Can you work these out from the model? Positions are in its coordinate system, mm. A direction names the side the tool comes from. Coordinates: 2 decimals unless noted, no trailing zeros. Loops run counter-clockwise (first coordinate to the right, second up) from the corner with the lowest first, then second, coordinate; pieces in that order, holes last. Notation, with made-up numbers: (17, 73.25) -> (34, 73.25) arc R20 cw to (34, 77.25) -> close; hole circle Ø7 at (3, -18). An arc over 180 degrees is marked (long way). Use one line per item in the form item = value. Start each with the question number.
(1) Imagine slicing it at A-A (y = -17.25). List the corners of the cut face in (x, z) for me (3 decimals), plus the area to 3 significant figures.
(2) Thinking about a two-plate mould opening in Z: for faces 5 (the flat face through (139.7, -9, 77)), 6 (the flat face through (129, -10, 104.775)), 7 (the flat face through (130, -10, 50.8)), which applies, released by +Z, released by -Z, zero draft, split by the parting line, or undercut?
(3) Imagine slicing it at C-C (z = 121). List the corners of the cut face in (x, y) for me (3 decimals), plus the area to 3 significant figures.
(4) I'm going to push flat-ended pins straight in: pin 1 (1 mm diameter, centred on y = -13.5, z = 128, fed in from +X) (3 decimals); pin 2 (9.5 mm diameter, centred on x = 131.5, y = -10, fed in from +Z) (3 decimals); pin 3 (5 mm diameter, centred on y = -15.5, z = 34, fed in from -X). Where does each tip first touch, or does it pass through?
(5) I need wall thicknesses on line 1 (X direction, y = -14.75, z = 110.5) (3 decimals); line 2 (X direction, y = -3.75, z = 34). Which ranges of each line are inside material? Lowest first, please. Write a range as [from, to].
(6) Imagine slicing it at B-B (x = 130.5). List the corners of the cut face in (y, z) for me (3 decimals).
(7) On a 3-axis mill with a long thin cutter (end or side, diameter ignored), from which of +Z, -Z, +X, -X, +Y, -Y can I reach the whole of each face in a straight line? I mean faces 1 (the flat face through (130.31, -9.66, 25.04)), 2 (the flat face through (22.225, -10, 128)), 3 (the flat face through (117.475, -10, 128)), 4 (the flat face through (9.39, -9.66, 25.04)). Say none if no direction works.
```python
from build123d import *

# Parameters (mm, degrees)
F0_W     = 139.7
F0_H     = 152.4
F1_DEPTH = 19.05
F2_W     = 22.225
F2_H     = 47.625
F3_DEPTH = 19.051
F6_DEPTH = 19.051


# Not quite as in the source:
# - a length typed as a fraction of an inch, garbled in the dataset ("3 / 203.2 mm" for 3/8 in), is restored
# - a pattern or mirror of a feature is missing from the dataset's text; its kind, count and spacing are read off the source's solid


with BuildPart() as f1:
    # F0 (on Front) → F1 (new body)
    with BuildSketch(Plane.XZ):
        with Locations((69.85, 76.2)):
            Rectangle(F0_W, F0_H)
    extrude(amount=F1_DEPTH)

    # F2 (on face) → F3 (cut, through all)
    with BuildSketch(Plane.XZ.offset(19.05)):
        with Locations((11.1125, 128.5875)):
            Rectangle(F2_W, F2_H)
    f3 = extrude(amount=-F3_DEPTH, mode=Mode.SUBTRACT)

    # F3_copies: F3 across plane
    add(f3.mirror(Plane(origin=(69.85, 0, 0), x_dir=(0, 0, 1), z_dir=(1, 0, 0))), mode=Mode.SUBTRACT)

    # F5 (on face) → F6 (cut, through all)
    with BuildSketch(Plane.XZ.offset(19.05)):
        Polygon((0, 50.8), (0, 0), (19.05, 50.8), align=None)
    f6 = extrude(amount=-F6_DEPTH, mode=Mode.SUBTRACT)

    # F6_copies: F6 across plane
    add(f6.mirror(Plane(origin=(69.85, 0, 0), x_dir=(0, 0, 1), z_dir=(1, 0, 0))), mode=Mode.SUBTRACT)


solid = f1.part
```
Worked out:
q1.outline = (0, 0) -> (139.7, 0) -> (120.65, 50.8) -> (139.7, 50.8) -> (139.7, 104.775) -> (117.475, 104.775) -> (117.475, 152.4) -> (22.225, 152.4) -> (22.225, 104.775) -> (0, 104.775) -> (0, 50.8) -> (19.05, 50.8) -> close
q1.area = 18,200 mm2
q2.face_5 = zero draft
q2.face_6 = released by +Z
q2.face_7 = undercut
q3.outline = (22.225, -19.05) -> (117.475, -19.05) -> (117.475, 0) -> (22.225, 0) -> close
q3.area = 1,810 mm2
q4.pin_1 = 117.475
q4.pin_2 = 104.775
q4.pin_3 = 11.81
q5.line_1 = [22.225, 117.475]
q5.line_2 = [12.75, 126.95]
q6.outline = (-19.05, 0) -> (0, 0) -> (0, 24.533) -> (-19.05, 24.533) -> close; (-19.05, 50.8) -> (0, 50.8) -> (0, 104.775) -> (-19.05, 104.775) -> close
q7.face_1 = +X, +Y, -Y
q7.face_2 = +Z, -X, +Y, -Y
q7.face_3 = +Z, +X, +Y, -Y
q7.face_4 = -X, +Y, -Y
